Model file for the job. Use its own axes, mm. Face numbers are marked on the shaded views. A direction names the side the tool comes from. Give positions to 0.01 mm unless a question says otherwise; leave off trailing zeros. Loops run counter-clockwise (first coordinate to the right, second up) from the corner with the lowest first, then second, coordinate; pieces in that order, holes last. Notation, with made-up numbers: (16, 20.5) - (36, 20.5) arc R28 cw to (36, 45.5) - close; hole circle Ø8 at (56.25, 15). An arc over 180 degrees is marked (long way). Use a Markdown table: item, result.
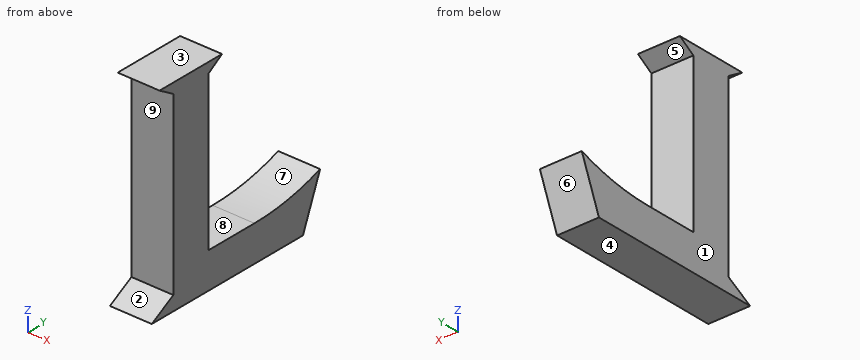
from build123d import *

# Parameters (mm, degrees)
F1_DEPTH = 12.05993
F3_DEPTH = 12.23708
F4_W     = 63.86287231
F4_H     = 63.649994554
F5_DEPTH = 2.13452
F6_R     = 49.0086529646
F6_W     = 63.86287231
F6_H     = 63.649994554
F7_DEPTH = 9.144


with BuildPart() as f1:
    # F0 (on Right) → F1 (new body)
    with BuildSketch(Plane.YZ):
        with BuildLine():
            Line((0, 4.1334182024), (-7.2379880522, 0))
            Line((-7.2379880522, 0), (43.5620119478, 0))
            Line((43.5620119478, 0), (49.3261106312, 14.2325060442))
            ThreePointArc((49.3261106312, 14.2325060442), (38.4755079225, 11.2506522164), (27.267575264, 10.2460244671))
            Line((27.267575264, 10.2460244671), (11.8531771004, 10.2460244671))
            Line((11.8531771004, 10.2460244671), (11.8531771004, 54.8946261406))
            Line((11.8531771004, 54.8946261406), (16.3711905479, 57.8180477023))
            Line((16.3711905479, 57.8180477023), (-4.6242829412, 57.8180477023))
            Line((-4.6242829412, 57.8180477023), (0, 54.9334182024))
            Line((0, 54.9334182024), (0, 4.1334182024))
        make_face()
    extrude(amount=F1_DEPTH)


with BuildPart() as f3:
    # F2 (on Right) → F3 (new body)
    with BuildSketch(Plane.YZ):
        Polygon((-8.8458675891, -1.5856656246), (-10.2534089237, -3.0272443658), (53.2465910763, -3.0272443658), (51.5569411218, -1.4188061468), align=None)
        Polygon((-10.2534089237, 60.4727556342), (-10.2534089237, -3.0272443658), (-8.8458675891, -1.5856656246), (-8.8458675891, 58.8171444833), align=None)
        Polygon((51.5569411218, -1.4188061468), (53.2465910763, -3.0272443658), (53.2465910763, 60.4727556342), (51.5569411218, 58.8171444833), align=None)
        Polygon((53.2465910763, 60.4727556342), (-10.2534089237, 60.4727556342), (-8.8458675891, 58.8171444833), (51.5569411218, 58.8171444833), align=None)
    extrude(amount=F3_DEPTH)


with BuildPart() as f5:
    # F4 (on Right) → F5 (new body)
    with BuildSketch(Plane.YZ):
        with Locations((21.525492426, 28.6787872901)):
            Rectangle(F4_W, F4_H)
    extrude(amount=-F5_DEPTH)

    # F6 (on face) → F7 (join)
    with BuildSketch(Plane(origin=(-2.13452, 0, 0), x_dir=(0, -1, 0), z_dir=(-1, 0, 0))):
        with Locations((-21.525492426, 28.6787872901)):
            Circle(F6_R)
        with Locations((-21.525492426, 28.6787872901)):
            Rectangle(F6_W, F6_H, mode=Mode.SUBTRACT)
    extrude(amount=-F7_DEPTH)


solid = f1.part
(1) 3-axis set-ups, long thin cutter, end or side, ignore diameter. For the marked faces 5, 6, 7, 8 and 9: which of +Z, -Z, +X, -X, +Y, -Y reach the whole face in a straight line?
Computed:
| item | result |
|---|---|
| face 5 | +X, -X, +Y |
| face 6 | -Z, +X, -X, +Y |
| face 7 | +Z, +X, -X |
| face 8 | +X, -X |
| face 9 | +X, -X, -Y |
(2) Slice it at C-C, the plane y = 23. Write the cut outline in (x, z), plus the area to 3 significant figures.
Computed:
| item | result |
|---|---|
| outline | (0, 0) - (12.06, 0) - (12.06, 10.25) - (0, 10.25) - close |
| area | 124 mm² |
(3) Slice it at B-B, the plane z = 47.5. Write the cut outline in (x, y).
Computed:
| item | result |
|---|---|
| outline | (0, 0) - (12.06, 0) - (12.06, 11.85) - (0, 11.85) - close |
(4) Slice it at A-A, the plane x = 4.5. Write the cut outline in (y, z), plus the area to 3 significant figures.
Computed:
| item | result |
|---|---|
| outline | (-7.24, 0) - (43.56, 0) - (49.33, 14.23) arc R63.02 cw to (27.27, 10.25) - (11.85, 10.25) - (11.85, 54.89) - (16.37, 57.82) - (-4.62, 57.82) - (0, 54.93) - (0, 4.13) - close |
| area | 1,090 mm² |
(5) Drill centre lines: probe 1 along Y at (x, z) = (5, 21.5); probe 2 along Z at (x, y) = (11, 18); probe 3 along Z at (x, y) = (1.75, 12.5). Where is each one in solid material? Low to high. Write a range as [from, to].
Computed:
| item | result |
|---|---|
| probe 1 | [0, 11.85] |
| probe 2 | [0, 10.25] |
| probe 3 | [0, 10.25], [55.31, 57.82] |
(6) Mould opens along Z. For the marked faces 1, 2, 3 and 4 say: pulls with the +Z half, pulls with the -Z half, needs draft (parallel to the pull), parting line crosses it, or undercut.
Computed:
| item | result |
|---|---|
| face 1 | needs draft |
| face 2 | undercut |
| face 3 | pulls with the +Z half |
| face 4 | pulls with the -Z half |
(7) Pin check, flat tips, straight feed: P1, Ø3, axis at x = 5.5, y = 1, coming from the -Z side; P2, Ø6, axis at x = 4, z = 35.5, coming from the -Y side; P3, Ø3.5, axis at x = 7, y = 21, coming from the +Z side; P4, Ø1.5, axis at x = 7.5, y = 33.5, coming from the +Z side. Stop position of each tip, or through.
Computed:
| item | result |
|---|---|
| P1 | z = 0 |
| P2 | y = 0 |
| P3 | z = 10.25 |
| P4 | z = 10.63 |
